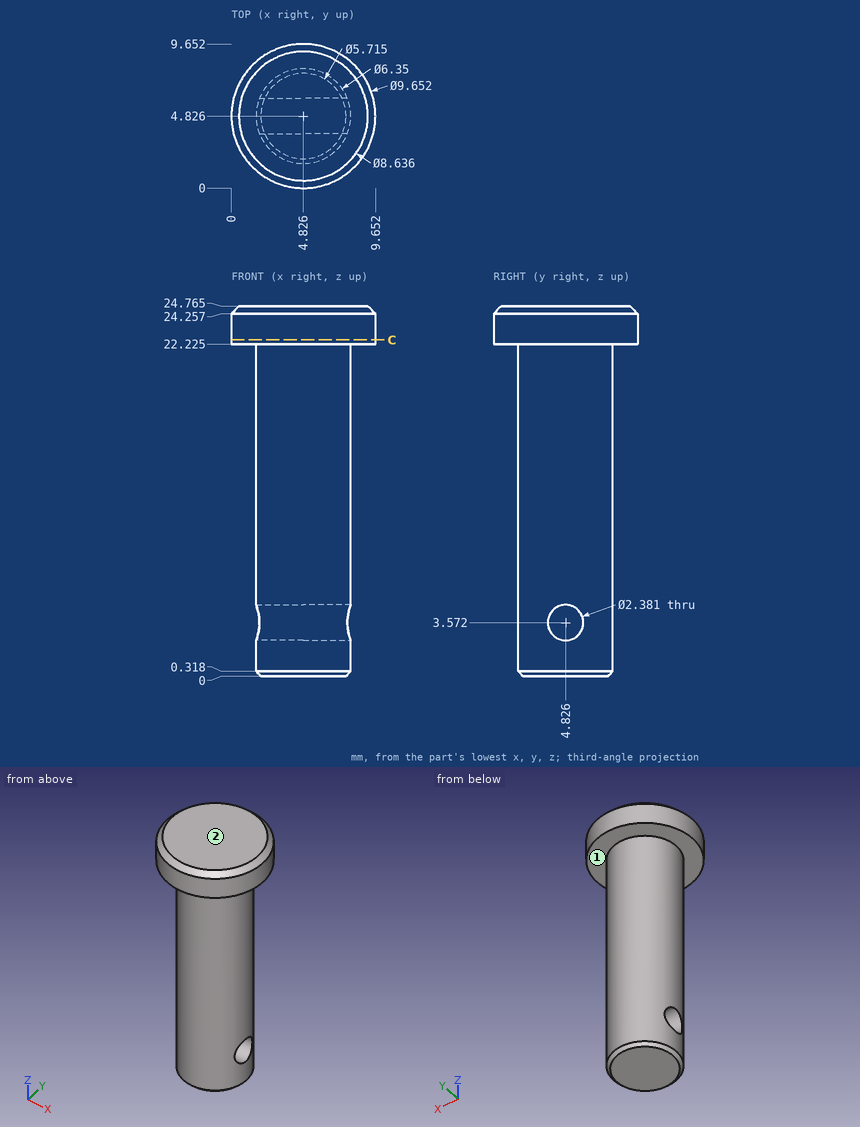
Design review of the part shown in the three views and the two pictorial views. Dimensions are in mm from the part's minimum x, y and z. A direction names the side the tool comes from. Round coordinates to 2 decimals unless told otherwise and drop trailing zeros. Loops run counter-clockwise (first coordinate to the right, second up) from the corner with the lowest first, then second, coordinate; pieces in that order, holes last. Notation, with made-up numbers: (24.25, -17.5) -> (53.25, -17.5) arc R21 cw to (53.25, 21.5) -> close; hole circle Ø10 at (42, 24). An arc over 180 degrees is marked (long way). Use one line per item in the form item = value. Start each with the question number.
Q1. We need section C-C on z = 22.5. Give the boundary of the cut face in (x, y) (1 decimal).
Q2. Machinability: for the marked faces 1 and 2, which of the approach directions +Z, -Z, +X, -X, +Y, -Y give a long, thin tool a straight path to every point of the face, cutting with its end or side? Answer none if there is none.
Q3. Wall thickness on line 1 along Z through (x, y) = (7.75, 7.5) (1 decimal); line 2 along Z through (x, y) = (4.5, 4) (1 decimal); line 3 along Y through (x, z) = (5.75, 3) (1 decimal): over which ranges is each line inside the solid? List them lowest first. Write a range as [from, to].
Q4. For pin 1 Ø1 at (x, z) = (3.5, 7) entering from +Y; pin 2 Ø1 at (y, z) = (6.5, 6.5) entering from -X (1 decimal); pin 3 Ø2 at (y, z) = (8.5, 11.5) entering from +X (1 decimal); pin 4 Ø1.4 at (y, z) = (4.83, 3.57) entering from -X, all flat-tipped, find the tip position at first contact; note any pin that passes through.
Calculated:
q1.outline = circle Ø9.7 at (4.8, 4.8)
q2.face_1 = -Z
q2.face_2 = +Z, +X, -X, +Y, -Y
q3.line_1 = [22.2, 24.8]
q3.line_2 = [0, 2.7], [4.4, 24.8]
q3.line_3 = [1.8, 3.8], [5.9, 7.9]
q4.pin_1 = 7.89
q4.pin_2 = 1.9
q4.pin_3 = 6.5
q4.pin_4 = through
